Drawing for the job (mm, zero at the part's lowest x, y, z). Give positions to 0.01 mm unless a question says otherwise; leave off trailing zeros. Loops run counter-clockwise (first coordinate to the right, second up) from the corner with the lowest first, then second, coordinate; pieces in that order, holes last. Notation, with made-up numbers: (18, 21) - (46, 21) arc R13 ccw to (46, 28) - close; hole circle Ø1 at (38, -34). An arc over 180 degrees is marked (long way). Return JSON: item names as keys, results as strings. Group by question number.
1) Slice it at B-B (x = 62.5). List the corners of the cut face in (y, z).
2) Slice it at A-A (y = 57.5). List the corners of the cut face in (x, z), and give its area (3 significant figures).
3) Slice it at C-C (z = 3.95). List the corners of the cut face in (x, y).
4) Slice it at D-D (x = 8). List the corners of the cut face in (y, z).
5) Drill centre lines: probe 1 along X at (y, z) = (57.5, 2.6); probe 2 along Y at (x, z) = (62.5, 2.75); probe 3 along X at (y, z) = (22.5, 4.4). Where is each one in solid material? Low to high. Write a range as from..to.
6) Drop flat-ended pins along their axis: pin 1 (2 mm diameter, centred on x = 25, z = 1, fed in from +Y); pin 2 (1.5 mm diameter, centred on x = 6, z = 2, fed in from -Y); pin 3 (1 mm diameter, centred on x = 81, z = 1.5, fed in from -Y). Give the stop position or say it passes through.
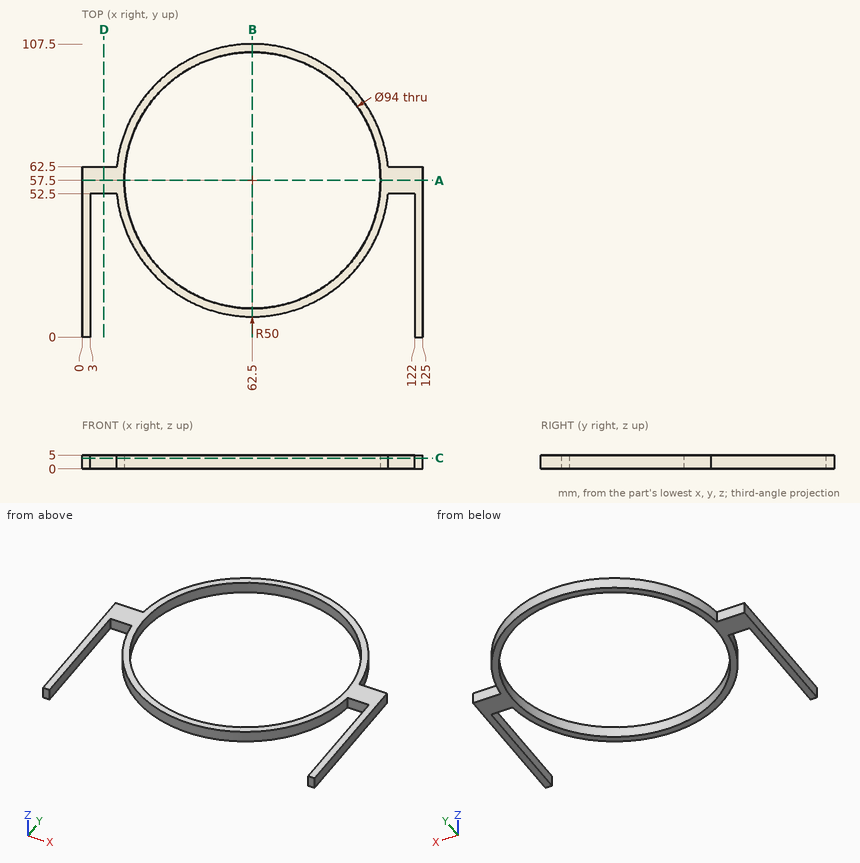
Results:
{
 "1": {"outline": "(7.5, 0) - (10.5, 0) - (10.5, 5) - (7.5, 5) - close; (104.5, 0) - (107.5, 0) - (107.5, 5) - (104.5, 5) - close"},
 "2": {"outline": "(0, 0) - (15.5, 0) - (15.5, 5) - (0, 5) - close; (109.5, 0) - (125, 0) - (125, 5) - (109.5, 5) - close", "area": "155 mm2"},
 "3": {"outline": "(0, 0) - (3, 0) - (3, 52.5) - (12.75, 52.5) arc R50 ccw to (112.25, 52.5) - (122, 52.5) - (122, 0) - (125, 0) - (125, 62.5) - (112.25, 62.5) arc R50 ccw to (12.75, 62.5) - (0, 62.5) - close; hole circle Ø94 at (62.5, 57.5)"},
 "4": {"outline": "(52.5, 0) - (62.5, 0) - (62.5, 5) - (52.5, 5) - close"},
 "5": {"probe 1": "0..15.5, 109.5..125", "probe 2": "7.5..10.5, 104.5..107.5", "probe 3": "0..3, 26.79..31.13, 93.87..98.21, 122..125"},
 "6": {"pin 1": "y = 91.67", "pin 2": "y = 52.5", "pin 3": "y = 10.85"}
}
